Build history of the part. All positions in model axes, mm. Give positions to 0.01 mm unless a question says otherwise; leave off trailing zeros. Order: outer loops, then holes, each group sorted by start corner. A loop starts at its lowest first (then second) coordinate and runs counter-clockwise, first axis right, second up. Notation, with made-up numbers: (72.25, 1) - (108.25, 1) arc R25 cw to (108.25, 17) - close; hole circle Ø8 at (4.25, -1). An arc over 180 degrees is marked (long way). One line per item, written item: value.
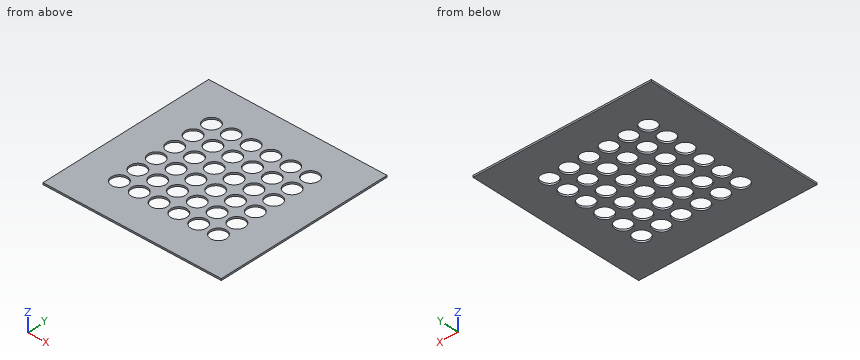
```python
from build123d import *

# Parameters (mm, degrees)
SKETCH048_W                     = 100
SKETCH048_H                     = 100
PAD018_DEPTH                    = 1
SKETCH049_R                     = 4.5
POCKET011_DEPTH                 = 283.850783
SKETCH049_LINEARPATTERN_2_R     = 4.5
POCKET011_LINEARPATTERN_2_DEPTH = 283.850783
SKETCH049_LINEARPATTERN_3_R     = 4.5
POCKET011_LINEARPATTERN_3_DEPTH = 283.850783
SKETCH049_LINEARPATTERN_4_R     = 4.5
POCKET011_LINEARPATTERN_4_DEPTH = 283.850783
SKETCH049_LINEARPATTERN_5_R     = 4.5
POCKET011_LINEARPATTERN_5_DEPTH = 283.850783
SKETCH049_LINEARPATTERN_6_R     = 4.5
POCKET011_LINEARPATTERN_6_DEPTH = 283.850783
LINEARPATTERN001_COUNT          = 6
LINEARPATTERN001_PITCH          = 11.111111


with BuildPart() as part:
    # Sketch048 → Pad018 (new body)
    with BuildSketch(Plane.XY):
        Rectangle(SKETCH048_W, SKETCH048_H)
    extrude(amount=PAD018_DEPTH)

    # Sketch049 → Pocket011 (cut, through all)
    with BuildSketch(Plane.XY):
        with Locations((-27.777778, 27.777778)):
            Circle(SKETCH049_R)
    pocket011 = extrude(amount=POCKET011_DEPTH, mode=Mode.SUBTRACT)

    # Sketch049 LinearPattern 2 → Pocket011 LinearPattern 2 (cut, through all)
    with BuildSketch(Plane(origin=(11.111111, 0, 0), x_dir=(1, 0, 0), z_dir=(0, 0, 1))):
        with Locations((-27.777778, 27.777778)):
            Circle(SKETCH049_LINEARPATTERN_2_R)
    pocket011_linearpattern_2 = extrude(amount=POCKET011_LINEARPATTERN_2_DEPTH, mode=Mode.SUBTRACT)

    # Sketch049 LinearPattern 3 → Pocket011 LinearPattern 3 (cut, through all)
    with BuildSketch(Plane(origin=(22.222222, 0, 0), x_dir=(1, 0, 0), z_dir=(0, 0, 1))):
        with Locations((-27.777778, 27.777778)):
            Circle(SKETCH049_LINEARPATTERN_3_R)
    pocket011_linearpattern_3 = extrude(amount=POCKET011_LINEARPATTERN_3_DEPTH, mode=Mode.SUBTRACT)

    # Sketch049 LinearPattern 4 → Pocket011 LinearPattern 4 (cut, through all)
    with BuildSketch(Plane(origin=(33.333333, 0, 0), x_dir=(1, 0, 0), z_dir=(0, 0, 1))):
        with Locations((-27.777778, 27.777778)):
            Circle(SKETCH049_LINEARPATTERN_4_R)
    pocket011_linearpattern_4 = extrude(amount=POCKET011_LINEARPATTERN_4_DEPTH, mode=Mode.SUBTRACT)

    # Sketch049 LinearPattern 5 → Pocket011 LinearPattern 5 (cut, through all)
    with BuildSketch(Plane(origin=(44.444444, 0, 0), x_dir=(1, 0, 0), z_dir=(0, 0, 1))):
        with Locations((-27.777778, 27.777778)):
            Circle(SKETCH049_LINEARPATTERN_5_R)
    pocket011_linearpattern_5 = extrude(amount=POCKET011_LINEARPATTERN_5_DEPTH, mode=Mode.SUBTRACT)

    # Sketch049 LinearPattern 6 → Pocket011 LinearPattern 6 (cut, through all)
    with BuildSketch(Plane(origin=(55.555556, 0, 0), x_dir=(1, 0, 0), z_dir=(0, 0, 1))):
        with Locations((-27.777778, 27.777778)):
            Circle(SKETCH049_LINEARPATTERN_6_R)
    pocket011_linearpattern_6 = extrude(amount=POCKET011_LINEARPATTERN_6_DEPTH, mode=Mode.SUBTRACT)

    # LinearPattern001: Pocket011, Pocket011 LinearPattern 2, Pocket011 LinearPattern 3, Pocket011 LinearPattern 4, Pocket011 LinearPattern 5, Pocket011 LinearPattern 6 ×6
    with Locations(*[(0, -i * LINEARPATTERN001_PITCH, 0) for i in range(1, LINEARPATTERN001_COUNT)]):
        add(pocket011, mode=Mode.SUBTRACT)
        add(pocket011_linearpattern_2, mode=Mode.SUBTRACT)
        add(pocket011_linearpattern_3, mode=Mode.SUBTRACT)
        add(pocket011_linearpattern_4, mode=Mode.SUBTRACT)
        add(pocket011_linearpattern_5, mode=Mode.SUBTRACT)
        add(pocket011_linearpattern_6, mode=Mode.SUBTRACT)


solid = part.part
```
(1) Pin check, flat tip, straight feed: P1, Ø7, axis at x = -27.78, y = -27.78, coming from the +Z side. Stop position of the tip, or through.
Completed:
P1: through
(2) Slice it at B-B, the plane x = 6.5. Give the cut face in (y, z), and give its area (3 significant figures).
Completed:
outline: (-50, 0) - (-32.18, 0) - (-32.18, 1) - (-50, 1) - close; (-23.38, 0) - (-21.07, 0) - (-21.07, 1) - (-23.38, 1) - close; (-12.27, 0) - (-9.96, 0) - (-9.96, 1) - (-12.27, 1) - close; (-1.16, 0) - (1.16, 0) - (1.16, 1) - (-1.16, 1) - close; (9.96, 0) - (12.27, 0) - (12.27, 1) - (9.96, 1) - close; (21.07, 0) - (23.38, 0) - (23.38, 1) - (21.07, 1) - close; (32.18, 0) - (50, 0) - (50, 1) - (32.18, 1) - close
area: 47.2 mm²
(3) Slice it at A-A, the plane y = 20. Give the cut face in (x, z).
Completed:
outline: (-50, 0) - (-30.8, 0) - (-30.8, 1) - (-50, 1) - close; (-24.75, 0) - (-19.69, 0) - (-19.69, 1) - (-24.75, 1) - close; (-13.64, 0) - (-8.58, 0) - (-8.58, 1) - (-13.64, 1) - close; (-2.53, 0) - (2.53, 0) - (2.53, 1) - (-2.53, 1) - close; (8.58, 0) - (13.64, 0) - (13.64, 1) - (8.58, 1) - close; (19.69, 0) - (24.75, 0) - (24.75, 1) - (19.69, 1) - close; (30.8, 0) - (50, 0) - (50, 1) - (30.8, 1) - close
(4) Slice it at C-C, the plane z = 0.2. Count the separate pieces of the cut face and the enclosed holes in it, and give its area (3 significant figures).
Completed:
separate pieces: 1
enclosed holes: 36
area: 7,710 mm²
